Source: CAD feature listing. Evaluate the final solid. Frame: model axes, mm. A direction names the side the tool comes from. Coordinates: 2 decimals unless noted, no trailing zeros. Loops run counter-clockwise (first coordinate to the right, second up) from the corner with the lowest first, then second, coordinate; pieces in that order, holes last.
```python
from build123d import *

# Parameters (mm, degrees)
F0_R     = 8.5
F1_DEPTH = 4
F2_R     = 5
F3_DEPTH = 100


with BuildPart() as f1:
    # F0 (on Top) → F1 (new body)
    with BuildSketch(Plane.XY):
        Circle(F0_R)
    extrude(amount=F1_DEPTH)

    # F2 (on Top) → F3 (join)
    with BuildSketch(Plane.XY):
        Circle(F2_R)
    extrude(amount=F3_DEPTH)

    # F4 (on Right) → F5 (revolve)
    with BuildSketch(Plane.YZ):
        with BuildLine():
            Line((3, 102), (0, 102))
            Line((0, 102), (0, 100))
            Line((0, 100), (5, 100))
            ThreePointArc((5, 100), (3.585786, 100.585786), (3, 102))
        make_face()
    revolve(axis=Axis((0, 0, 101), (0, 0, -1)))

    # F6 (on Right) → F7 (revolve)
    with BuildSketch(Plane.YZ):
        with BuildLine():
            Line((0, 104), (0, 102))
            Line((0, 102), (3, 102))
            ThreePointArc((3, 102), (2.414214, 103.414214), (1, 104))
            Line((1, 104), (0, 104))
        make_face()
    revolve(axis=Axis((0, 0, 103), (0, 0, 1)))


solid = f1.part
```
Q1. Section query B-B on z = 55.5. Return the cut outline in (x, y).
Q2. Section query C-C on x = -6. Return the cut outline in (y, z).
Q3. Section query A-A on y = -7.5. Return the cut outline in (x, z).
Q4. First-contact query: pin 1 Ø5 at (y, z) = (2.5, 64.5) entering from -X; pin 2 Ø6 at (x, y) = (0.5, 4.5) entering from +Z; pin 3 Ø8 at (x, z) = (-2, 34) entering from -Y. Flat tips, straight axial feed; report the tip coordinate or a pass-through.
Q5. Reachability of faces 1 (the flat face through (0, 0, 104)), 2 (the flat face through (4, -4, 4)) from +Z, -Z, +X, -X, +Y, -Y: full face, straight path, thin tool, end or side. Return the list, or none.
Q6. Material intervals for line 1 along Z through (x, y) = (-1.25, -6.5); line 2 along X through (y, z) = (0.25, 81); line 3 along Y through (x, z) = (-4, 13.5), sorted ascending.
Resolved:
1. outline: circle Ø10 at (0, 0)
2. outline: (-6.02, 0) - (6.02, 0) - (6.02, 4) - (-6.02, 4) - close
3. outline: (-4, 0) - (4, 0) - (4, 4) - (-4, 4) - close
4. pin 1: stops at x = -5
4. pin 2: stops at z = 103.93
4. pin 3: stops at y = -5
5. face 1: +Z, +X, -X, +Y, -Y
5. face 2: +Z
6. line 1: z = 0 to 4
6. line 2: x = -4.99 to 4.99
6. line 3: y = -3 to 3
